Read the model definition and answer for the solid it produces. Units are mm, in the model's axes. A direction names the side the tool comes from. Give positions to 0.01 mm unless a question says otherwise; leave off trailing zeros. Order: outer loops, then holes, each group sorted by start corner. A loop starts at its lowest first (then second) coordinate and runs counter-clockwise, first axis right, second up. Notation, with made-up numbers: M 39.25,30 L 49.25,30 A33 ccw 49.25,58 Z; hole C 69,4.25 d4. An arc over 180 degrees is marked long. One line per item, written item: value.
from build123d import *

# Parameters (mm, degrees)
SKETCH1_R           = 3.175
SKETCH1_R_2         = 2.4892
BOSS_EXTRUDE1_DEPTH = 6.858
SKETCH2_R           = 4.064
BOSS_EXTRUDE2_DEPTH = 1.905
SKETCH3_R           = 2.4892
CUT_EXTRUDE1_DEPTH  = 11.479616453


with BuildPart() as part:
    # Sketch1 → Boss-Extrude1 (new body)
    with BuildSketch(Plane(origin=(0, 0, 0), x_dir=(1, 0, 0), z_dir=(0, 1, 0))):
        with Locations(Location((0, 0, 0), (0, 0, 270))):
            Circle(SKETCH1_R)
        with Locations(Location((0, 0, 0), (0, 0, 270))):
            Circle(SKETCH1_R_2, mode=Mode.SUBTRACT)
    extrude(amount=BOSS_EXTRUDE1_DEPTH)

    # Sketch2 → Boss-Extrude2 (add)
    with BuildSketch(Plane.XZ):
        with Locations(Location((0, 0, 0), (0, 0, 90))):
            Circle(SKETCH2_R)
    extrude(amount=BOSS_EXTRUDE2_DEPTH)

    # Sketch3 → Cut-Extrude1 (cut, through all)
    with BuildSketch(Plane.XZ.offset(1.905)):
        with Locations(Location((0, 0, 0), (0, 0, 270))):
            Circle(SKETCH3_R)
    extrude(amount=-CUT_EXTRUDE1_DEPTH, mode=Mode.SUBTRACT)


solid = part.part
1) Find section C-C, the plane z = 3. Write down the section's boundary in (x, y) (3 decimals).
Reported:
outline: M -2.742,-1.905 L 2.742,-1.905 L 2.742,0 L 1.04,0 L 1.04,6.858 L -1.04,6.858 L -1.04,0 L -2.742,0 Z
2) Each of these flat-tipped pins is pushed along its axis until it touches: pin 1 Ø1 at (x, y) = (-2.5, 2) entering from +Z; pin 2 Ø3 at (y, z) = (0.5, 2) entering from +X; pin 3 Ø1 at (y, z) = (-0.5, 3) entering from +X. Where does it stop, or does it pass through?
Reported:
pin 1: stops at z = 2.47
pin 2: stops at x = 4.02
pin 3: stops at x = 3.2
3) Determine the mould class of faces 3 (the face through (3.967, -0.939, -0.881)), 4 (the face through (2, -1.905, -2)), 5 (the face through (0.748, 2.415, -2.374)) for opening direction Z: +Z half, -Z half, draft (parallel to the pull), parting line (faces both ways), or undercut.
Reported:
face 3: parting line
face 4: draft
face 5: undercut
4) Find section B-B, the plane x = 0. Write down the section's boundary in (y, z) (3 decimals).
Reported:
outline: M -1.905,-4.064 L 0,-4.064 L 0,-3.175 L 6.858,-3.175 L 6.858,-2.489 L -1.905,-2.489 Z; M -1.905,2.489 L 6.858,2.489 L 6.858,3.175 L 0,3.175 L 0,4.064 L -1.905,4.064 Z
5) Find section D-D, the plane y = 6. Write down the section's boundary in (x, z) (3 decimals).
Reported:
outline: C 0,0 d6.35; hole C 0,0 d4.978
6) Consider probe 1 along X at (y, z) = (0.25, 0) (3 decimals); probe 2 along Y at (x, z) = (-3.5, -0.75) (3 decimals); probe 3 along X at (y, z) = (4.5, 2.25). Determine where each line is inside the solid, lowest interval first.
Reported:
probe 1: x = -3.175 to -2.489, 2.489 to 3.175
probe 2: y = -1.905 to 0
probe 3: x = -2.24 to -1.06, 1.06 to 2.24
7) Which of the six approach directions +Z, -Z, +X, -X, +Y, -Y give full straight-line access (tool end or side, diameter ignored) to faces 1 (the face through (-2, 6.858, -2)), 2 (the face through (-1.93, 3.38, -2.52))?
Reported:
face 1: +Z, -Z, +X, -X, +Y
face 2: +Y
8) Find section A-A, the plane z = 0. Write down the section's boundary in (x, y) (3 decimals).
Reported:
outline: M -4.064,-1.905 L -2.489,-1.905 L -2.489,6.858 L -3.175,6.858 L -3.175,0 L -4.064,0 Z; M 2.489,-1.905 L 4.064,-1.905 L 4.064,0 L 3.175,0 L 3.175,6.858 L 2.489,6.858 Z
